Geometry: final body of the model. Coordinates: model frame, mm. Round coordinates to 2 decimals unless told otherwise and drop trailing zeros. Loops run counter-clockwise (first coordinate to the right, second up) from the corner with the lowest first, then second, coordinate; pieces in that order, holes last. Notation, with made-up numbers: (26.5, -35.5) - (42.5, -35.5) arc R20 cw to (42.5, -3.5) - close; hole circle Ø2 at (-20, 50). An arc over 180 degrees is marked (long way). Answer in a Markdown table with one row per item. Add a question column.
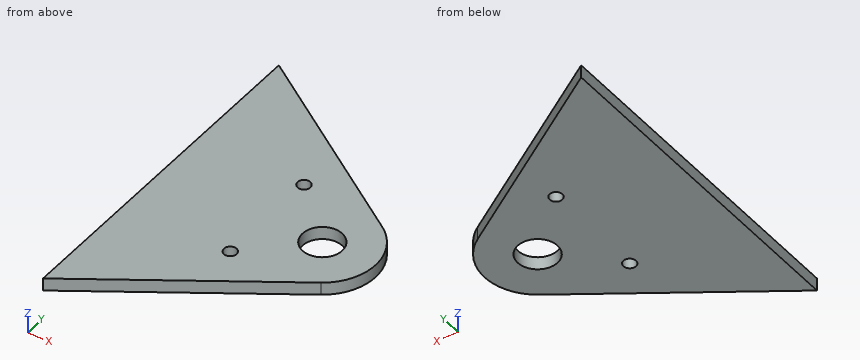
Autodesk Inventor part; units mm, degrees
ref_plane "YZ Plane" through (0, 0, 0) normal (1, 0, 0) x (0, 1, 0)
ref_plane "XZ Plane" through (0, 0, 0) normal (0, 1, 0) x (-1, 0, 0)
ref_plane "XY Plane" through (0, 0, 0) normal (0, 0, 1) x (1, 0, 0)
sketch "Sketch1" plane through (0, 0, 0) normal (0, 0, 1) x (1, 0, 0)
  circle A0 centre (21.9255, 0) radius 6.5 construction
  arc A1 (28.8018, -10.4387) -> (28.8018, 10.4387) centre (21.9255, 0) ccw
  line L0 (-16.0745, -40) -> (28.8018, -10.4387)
  line L1 (28.8018, 10.4387) -> (-16.0745, 40)
  line L2 (-16.0745, 40) -> (-16.0745, 17)
  line L3 (-16.0745, -17) -> (-16.0745, -40)
  line L4 (-16.0745, -40) -> (-16.0745, 40)
  circle A2 centre (21.9255, 0) radius 4.675
  circle A3 centre (8.9255, -12.5) radius 1.5
  line L5 (-16.0745, 0) -> (34.4255, 0) construction
  circle A4 centre (8.9255, 12.5) radius 1.5
  point P0 (0, 0)
  dimension "d0" = 9.35
  dimension "d1" = 3
  dimension "d2" = 25
  dimension "d3" = 12.5
extrude "Extrusion1" add sketch "Sketch1" along normal blind 3
properties part number "Bearing lockers"
1) Section B-B, the plane z = 2.1. Give the number of separate pieces and of enclosed holes in the cut face, and give its area (3 significant figures).
2) Section D-D, the plane x = -11. Return the cut outline in (y, z), and give its area (3 significant figures).
3) Section A-A, the plane y = 0. Return the cut outline in (x, z), and give its area (3 significant figures).
4) Section C-C, the plane y = 12.5. Return the cut outline in (x, z).
5) Material intervals for line 1 along Y through (x, z) = (26, 1.7); line 2 along X through (y, z) = (-4, 1.15); line 3 along Y through (x, z) = (-10, 2.35), sorted ascending. Write a range as from..to.
6) Contact query for a flat-ended pin moving along its axis: pin 1 Ø3 at (x, y) = (16, 21.5) entering from -Z. Output: stop coordinate, or through.
Evaluation:
| question | item | result |
|---|---|---|
| 1 | separate pieces | 1 |
| 1 | enclosed holes | 3 |
| 1 | area | 2,260 mm² |
| 2 | outline | (-36.66, 0) - (36.66, 0) - (36.66, 3) - (-36.66, 3) - close |
| 2 | area | 220 mm² |
| 3 | outline | (-16.07, 0) - (17.25, 0) - (17.25, 3) - (-16.07, 3) - close; (26.6, 0) - (34.43, 0) - (34.43, 3) - (26.6, 3) - close |
| 3 | area | 123 mm² |
| 4 | outline | (-16.07, 0) - (7.43, 0) - (7.43, 3) - (-16.07, 3) - close; (10.43, 0) - (25.67, 0) - (25.67, 3) - (10.43, 3) - close |
| 5 | line 1 | y = -12.28..-2.29, 2.29..12.28 |
| 5 | line 2 | x = -16.07..19.51, 24.35..33.77 |
| 5 | line 3 | y = -36..36 |
| 6 | pin 1 | passes through |
